from build123d import *

# Parameters (mm, degrees)
SKETCH_1_R               = 6
EXTRUDE_1_DEPTH          = 10
SKETCH_2_R               = 10
EXTRUDE_2_DEPTH          = 6
SKETCH_2_3_R             = 10
EXTRUDE_3_DEPTH          = 32
CUT_EXTRUDE_1_REACH      = 94.136
CUT_EXTRUDE_1_END_RADIUS = 10
SKETCH_3_R               = 8


with BuildPart() as part:
    # 草图1 → 凸台-拉伸1 (new body)
    with BuildSketch(Plane.XY):
        with BuildLine():
            Line((-31, -50), (-12, -50))
            Line((-12, -50), (-12, -44))
            Line((-12, -44), (12, -44))
            Line((12, -44), (12, -50))
            Line((12, -50), (31, -50))
            ThreePointArc((31, -50), (38.778174593, -46.778174593), (42, -39))
            Line((42, -39), (42, 0))
            Line((42, 0), (-42, 0))
            Line((-42, 0), (-42, -39))
            ThreePointArc((-42, -39), (-38.778174593, -46.778174593), (-31, -50))
        make_face()
        with Locations((31, -39)):
            Circle(SKETCH_1_R, mode=Mode.SUBTRACT)
        with Locations(Location((-31, -39, 0), (0, 0, 180))):
            Circle(SKETCH_1_R, mode=Mode.SUBTRACT)
    extrude(amount=EXTRUDE_1_DEPTH)

    # 草图2 → 凸台-拉伸2 (add)
    with BuildSketch(Plane(origin=(0, 0, 0), x_dir=(1, 0, 0), z_dir=(0, 1, 0))):
        with BuildLine():
            Line((32, 0), (19.255885515, 45.404708412))
            ThreePointArc((19.255885515, 45.404708412), (0, 60), (-19.255885515, 45.404708412))
            Line((-19.255885515, 45.404708412), (-32, 0))
            Line((-32, 0), (32, 0))
        make_face()
        with Locations(Location((0, 40, 0), (0, 0, 180))):
            Circle(SKETCH_2_R, mode=Mode.SUBTRACT)
    extrude(amount=-EXTRUDE_2_DEPTH)

    # 草图2<3> → 凸台-拉伸3 (add)
    with BuildSketch(Plane(origin=(0, 0, 0), x_dir=(1, 0, 0), z_dir=(0, 1, 0))):
        with BuildLine():
            ThreePointArc((3, 20.226280067), (16.802363629, 29.151932131), (19.255885515, 45.404708412))
            ThreePointArc((19.255885515, 45.404708412), (16.936067955, 50.638120239), (13.228756555, 55))
            Line((13.228756555, 55), (-13.228756555, 55))
            ThreePointArc((-13.228756555, 55), (-16.936067955, 50.638120239), (-19.255885515, 45.404708412))
            ThreePointArc((-19.255885515, 45.404708412), (-16.802363629, 29.151932131), (-3, 20.226280067))
            Line((-3, 20.226280067), (-3, 0))
            Line((-3, 0), (3, 0))
            Line((3, 0), (3, 20.226280067))
        make_face()
        with Locations(Location((0, 40, 0), (0, 0, 180))):
            Circle(SKETCH_2_3_R, mode=Mode.SUBTRACT)
    extrude(amount=-EXTRUDE_3_DEPTH)

    # 切除-拉伸1: up to this cylinder (the profile starts outside it)
    cut_extrude_1_end = Plane(origin=(0, -19, -40), z_dir=(0, 1, 0)) * Cylinder(CUT_EXTRUDE_1_END_RADIUS, 209.272, mode=Mode.PRIVATE)
    # 草图3 → 切除-拉伸1 (cut, up to the surface)
    with BuildSketch(Plane(origin=(0, 0, -55), x_dir=(-1, 0, 0), z_dir=(0, 0, -1)), mode=Mode.PRIVATE) as cut_extrude_1_sk1:
        with Locations((0, -19)):
            Circle(SKETCH_3_R)
    cut_extrude_1_tool1 = extrude(cut_extrude_1_sk1.sketch, amount=-CUT_EXTRUDE_1_REACH, mode=Mode.PRIVATE) - cut_extrude_1_end
    add(cut_extrude_1_tool1.solids().sort_by_distance((0, -19, -55))[0], mode=Mode.SUBTRACT)


solid = part.part
The listing builds one solid part. Answer for the finished solid, in the listing's coordinates (mm). A direction names the side the tool comes from. Coordinates: 2 decimals unless noted, no trailing zeros. Order: outer loops, then holes, each group sorted by start corner. A loop starts at its lowest first (then second) coordinate and runs counter-clockwise, first axis right, second up.
Q1. A cutting plane is placed at B-B, the plane x = 0. Write down the section's boundary in (y, z).
Q2. Consider line 1 (Y direction, x = 31, z = 4); line 2 (Z direction, x = 0, y = -14); line 3 (Y direction, x = -10, z = -35.5). Determine where each line is inside the solid, lowest interval first.
Q3. A cutting plane is placed at C-C, the plane z = -40. Write down the section's boundary in (x, y), and give its area (3 significant figures).
Q4. A cutting plane is placed at D-D, the plane y = -19. Write down the section's boundary in (x, z), and give its area (3 significant figures).
Q5. For a pull along X with two mould halves and no side action, classify faces 1 (the face through (1.302, -15.776, -30.085)), 2 (the face through (-18, -6, -13)), 3 (the face through (12, -47, 5)), 4 (the face through (3, -19, -10)) as pulls with the +X half, pulls with the -X half, needs draft (parallel to the pull), parting line crosses it, or undercut.
Q6. Given P1, Ø4, axis at y = -23, z = -20, coming from the -X side; P2, Ø1.5, axis at y = -31.5, z = -50.5, coming from the -X side; P3, Ø14.5, axis at x = 0, y = -19, coming from the -Z side, each flat-ended and moving along its own axis, determine where each tip first touches the part or whether it passes through.
Q7. A cutting plane is placed at A-A, the plane y = -30. Write down the section's boundary in (x, z), and give its area (3 significant figures).
Q8. Which of the six approach directions +Z, -Z, +X, -X, +Y, -Y give full straight-line access (tool end or side, diameter ignored) to faces 5 (the face through (0, -32, -28)), 6 (the face through (0, -44, 5)), 7 (the face through (-10.02, -15.78, -22.69)), 8 (the face through (17, -6, -13))?
Answers follow:
1. outline: (-44, 0) - (-32, 0) - (-32, -30) - (0, -30) - (0, 10) - (-44, 10) - close; (-32, -55) - (-27, -55) - (-27, -50) - (-32, -50) - close; (-11, -55) - (-6, -55) - (-6, -60) - (0, -60) - (0, -50) - (-11, -50) - close
2. line 1: y = -50 to -45, -33 to 0
2. line 2: z = -30 to 10
2. line 3: y = -32 to 0
3. outline: (-20.77, -6) - (-20, -6) - (-20, -32) - (-10, -32) - (-10, 0) - (-20.77, 0) - close; (10, -32) - (20, -32) - (20, -6) - (20.77, -6) - (20.77, 0) - (10, 0) - close
3. area: 649 mm2
4. outline: (-42, 0) - (-3, 0) - (-3, -20.23) arc R20 ccw to (-13.23, -55) - (-8, -55) - (-8, -46) arc R10 cw (long way) to (8, -46) - (8, -55) - (13.23, -55) arc R20 ccw to (3, -20.23) - (3, 0) - (42, 0) - (42, 10) - (-42, 10) - close
4. area: 1,710 mm2
5. face 1: undercut
5. face 2: needs draft
5. face 3: undercut
5. face 4: pulls with the +X half
6. P1: stops at x = -8.72
6. P2: stops at x = -17.46
6. P3: stops at z = -33.11
7. outline: (-42, 0) - (-3, 0) - (-3, -20.23) arc R20 ccw to (-13.23, -55) - (13.23, -55) arc R20 ccw to (3, -20.23) - (3, 0) - (42, 0) - (42, 10) - (-42, 10) - close; hole circle Ø20 at (0, -40)
7. area: 1,810 mm2
8. face 5: -Z, +X, -X, -Y
8. face 6: +Z, -Z, -Y
8. face 7: -Y
8. face 8: +X, -Y
